```python
from build123d import *

# Parameters (mm, degrees)
SALIENTE_EXTRUIR1_DEPTH = 10
CORTAR_EXTRUIR1_DEPTH   = 10


with BuildPart() as part:
    # Croquis2 → Saliente-Extruir1 (new body)
    with BuildSketch(Plane.XY):
        with BuildLine():
            Line((-19.5, 0), (-29.7, 0))
            Line((-29.7, 0), (-29.7, 55))
            Line((-29.7, 55), (29.7, 55))
            Line((29.7, 55), (29.7, 0))
            Line((29.7, 0), (19.5, 0))
            Line((19.5, 0), (19.5, 30.5))
            ThreePointArc((19.5, 30.5), (0, 50), (-19.5, 30.5))
            Line((-19.5, 30.5), (-19.5, 0))
        make_face()
    extrude(amount=SALIENTE_EXTRUIR1_DEPTH)

    # Croquis3 → Cortar-Extruir1 (cut)
    with BuildSketch(Plane.XZ):
        Polygon((19.5, 5), (19.5, 8.6), (24.7, 8.6), (24.7, 1.4), (19.5, 1.4), align=None)
        Polygon((-24.7, 1.4), (-19.5, 1.4), (-19.5, 5), (-19.5, 8.6), (-24.7, 8.6), align=None)
    extrude(amount=-CORTAR_EXTRUIR1_DEPTH, mode=Mode.SUBTRACT)


solid = part.part
```
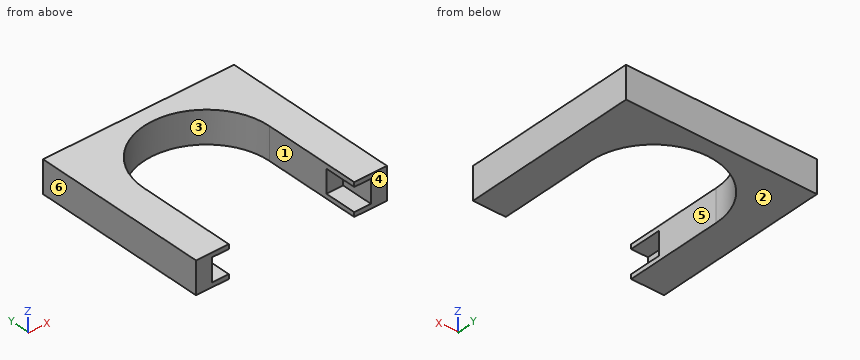
Source: CAD feature listing. Evaluate the final solid. Frame: model axes, mm. Face numbers are marked on the shaded views. A direction names the side the tool comes from. Coordinates: 2 decimals unless noted, no trailing zeros. Loops run counter-clockwise (first coordinate to the right, second up) from the corner with the lowest first, then second, coordinate; pieces in that order, holes last. Notation, with made-up numbers: M 57.5,25.5 L 108.5,25.5 A26 ccw 108.5,44.5 Z; hole C 24.25,6.5 d11. An arc over 180 degrees is marked long. Use a Markdown table: item, result. Add a question column.
Q1. Section query A-A, the plane y = 5. Return loops of the section in (x, z).
Q2. Material intervals for L1, parallel to X at y = 4.5, z = 5.5; L2, parallel to X at y = 27, z = 7; L3, parallel to Y at x = -22, z = 3, sorted ascending.
Q3. First-contact query: pin 1 (3 mm diameter, centred on x = 22.5, z = 3, fed in from -Y). Flat tip, straight axial feed; report the tip coordinate or a pass-through.
Q4. Draft query along X for the marked faces 3, 4, 5 and 6. Return one class per face: pulls with the +X half, pulls with the -X half, needs draft (parallel to the pull), parting line crosses it, or undercut.
Q5. Section query D-D, the plane y = 32. Return loops of the section in (x, z), and give its area (3 significant figures).
Q6. Access query for the marked faces 1 and 2. Directions: +Z, -Z, +X, -X, +Y, -Y. A direction counts if a zero-diameter tool reaches every point of the face in a straight line with its end or side. Return the directions, or none.
Q7. Section query B-B, the plane z = 2.5. Return loops of the section in (x, y).
Q8. Section query C-C, the plane x = 0. Return loops of the section in (y, z).
Result:
| question | item | result |
|---|---|---|
| 1 | outline | M -29.7,0 L -19.5,0 L -19.5,1.4 L -24.7,1.4 L -24.7,8.6 L -19.5,8.6 L -19.5,10 L -29.7,10 Z; M 19.5,0 L 29.7,0 L 29.7,10 L 19.5,10 L 19.5,8.6 L 24.7,8.6 L 24.7,1.4 L 19.5,1.4 Z |
| 2 | L1 | x = -29.7 to -24.7, 24.7 to 29.7 |
| 2 | L2 | x = -29.7 to -19.5, 19.5 to 29.7 |
| 2 | L3 | y = 10 to 55 |
| 3 | pin 1 | stops at y = 10 |
| 4 | face 3 | undercut |
| 4 | face 4 | needs draft |
| 4 | face 5 | undercut |
| 4 | face 6 | pulls with the -X half |
| 5 | outline | M -29.7,0 L -19.44,0 L -19.44,10 L -29.7,10 Z; M 19.44,0 L 29.7,0 L 29.7,10 L 19.44,10 Z |
| 5 | area | 205 mm2 |
| 6 | face 1 | +Z, -Z, -Y |
| 6 | face 2 | -Z, +X, -X, +Y, -Y |
| 7 | outline | M -29.7,0 L -24.7,0 L -24.7,10 L -19.5,10 L -19.5,30.5 A19.5 cw 19.5,30.5 L 19.5,10 L 24.7,10 L 24.7,0 L 29.7,0 L 29.7,55 L -29.7,55 Z |
| 8 | outline | M 50,0 L 55,0 L 55,10 L 50,10 Z |
